Job drawing, mm, ordinate dimensions from the low corner. One solid piece. A direction names the side the tool comes from. Give positions to 0.01 mm unless a question says otherwise; leave off trailing zeros. Loops run counter-clockwise (first coordinate to the right, second up) from the corner with the lowest first, then second, coordinate; pieces in that order, holes last. Notation, with made-up numbers: M 0,-10 L 35,-10 A30 cw 35,17 Z; hole C -6.5,83 d7. An arc over 180 degrees is marked long. Answer in a Markdown table with one row per item.
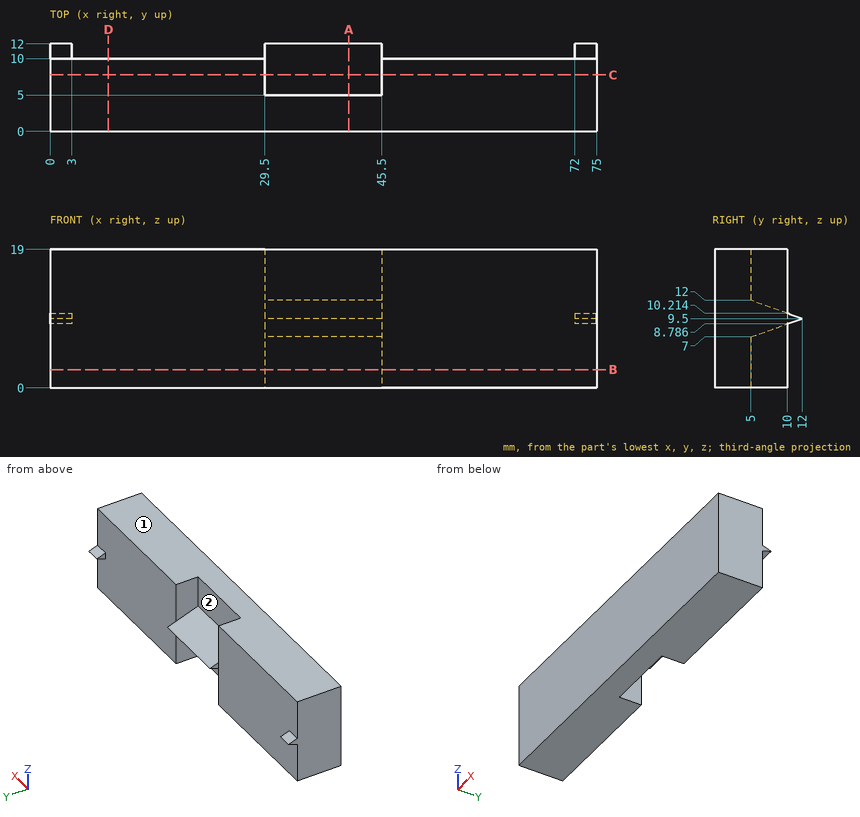
(1) Saw through at A-A (x = 41). Write the cut outline in (y, z).
Recorded:
| item | result |
|---|---|
| outline | M 0,0 L 5,0 L 5,7 L 12,9.5 L 5,12 L 5,19 L 0,19 Z |
(2) Pin check, flat tips, straight feed: pin 1 Ø1.5 at (x, z) = (55.5, 4) entering from +Y; pin 2 Ø4 at (y, z) = (8, 15) entering from -X; pin 3 Ø3.5 at (x, z) = (36, 15.5) entering from +Y. Stop position of each tip, or through.
Recorded:
| item | result |
|---|---|
| pin 1 | stops at y = 10 |
| pin 2 | stops at x = 0 |
| pin 3 | stops at y = 5 |
(3) Saw through at B-B (z = 2.5). Write the cut outline in (x, y), plus the area to 3 significant figures.
Recorded:
| item | result |
|---|---|
| outline | M 0,0 L 75,0 L 75,10 L 45.5,10 L 45.5,5 L 29.5,5 L 29.5,10 L 0,10 Z |
| area | 670 mm^2 |
(4) Saw through at C-C (y = 7.75). Write the cut outline in (x, z).
Recorded:
| item | result |
|---|---|
| outline | M 0,0 L 29.5,0 L 29.5,7.98 L 45.5,7.98 L 45.5,0 L 75,0 L 75,19 L 45.5,19 L 45.5,11.02 L 29.5,11.02 L 29.5,19 L 0,19 Z |
(5) Drill centre lines: line 1 along X through (y, z) = (8, 4.25); line 2 along Y through (x, z) = (20.5, 9.25); line 3 along Z through (x, y) = (36, 11.5). Where is each one in solid material? Low to high.
Recorded:
| item | result |
|---|---|
| line 1 | x = 0 to 29.5, 45.5 to 75 |
| line 2 | y = 0 to 10 |
| line 3 | z = 9.32 to 9.68 |
(6) Which spindle directions (+Z, -Z, +X, -X, +Y, -Y) get a long thin tool onto all of the face, cutting with end or side? Do the marked faces 1 and 2. Say none if no direction does.
Recorded:
| item | result |
|---|---|
| face 1 | +Z, +X, -X, +Y, -Y |
| face 2 | +Z, +Y |
(7) Saw through at D-D (x = 8). Write the cut outline in (y, z), plus the area to 3 significant figures.
Recorded:
| item | result |
|---|---|
| outline | M 0,0 L 10,0 L 10,19 L 0,19 Z |
| area | 190 mm^2 |
